Autodesk Inventor part; units mm, degrees
ref_plane "Start Plane" through (0, 0, -31.4468) normal (0, 0, 1) x (1, 0, 0)
ref_plane "End Plane" through (0, 0, 1160.255) normal (0, 0, 1) x (1, 0, 0)
ref_plane "Work Plane4" through (-6.5041, 0, 1155.5322) normal (0.2588, 0, 0.9659) x (0.9659, 0, -0.2588)
ref_plane "Start Plane" through (0, 0, -31.4468) normal (0, 0, 1) x (1, 0, 0)
ref_plane "End Plane" through (0, 0, 1160.255) normal (0, 0, 1) x (1, 0, 0)
sketch "Sketch" plane through (0, 0, 0) normal (0, 0, 1) x (1, 0, 0)
  circle A0 centre (0, 0) radius 20.447
  circle A1 centre (0, 0) radius 24.13
  dimension "d0" = 48.26
  dimension "d1" = 3.683
extrude "Body" add sketch "Sketch" along normal up to surface (1191.7019 mm away) from surface at -31.4468
sketch "Sketch3" plane through (0, 0, 0) normal (0, 0, 1) x (1, 0, 0)
  line L0 (0, 0) -> (10, 0)
ref_plane "Work Plane3" through (0, 0, 0) normal (0, -1, 0) x (1, 0, 0)
ref_plane "Work Plane4" through (-6.5041, 0, 1155.5322) normal (0.2588, 0, 0.9659) x (0.9659, 0, -0.2588)
split "Split1" plane through (-6.5041, 0, 1155.5322) removes the side toward (0.2588, 0, 0.9659)
ref_plane "Work Plane5" through (-982.5186, 0, 238.2838) normal (-0.2588, 0, -0.9659) x (-0.9659, 0, 0.2588)
split "Split2" plane through (-982.5186, 0, 238.2838) removes the side toward (-0.2588, 0, -0.9659)
sketch "Sketch4" plane through (0, 0, 0) normal (0, -1, 0) x (1, 0, 0)
  line L0 (-2, -31.4468) -> (12, -31.4468)
  line L1 (-2, 1160.255) -> (12, 1160.255)
  dimension "d7" = 1191.7018
equation "\"d0\" = G_H"
equation "\"d1\" = G_T"
equation "\"d2\" = G_L"
equation "\"G_H\" = 48.26"
equation "\"G_T\" = 3.683"
equation "\"G_L\" = d7"
equation "\"G_OFFSET_START\" = 31.44683"
equation "\"G_OFFSET_END\" = -19.55088"
equation "\"d4\" = -G_OFFSET_START"
equation "\"d5\" = G_OFFSET_END + B_L"
equation "\"B_L\" = 1179.8059"
properties part number "ANSI - 1 1/2 x 0.145 - 46.917" material "Steel, Mild"
Design review of the part built by this model. Coordinates are the model's own, in mm. Coordinates: 2 decimals unless noted, no trailing zeros. Write each loop counter-clockwise with the first axis right and the second up, starting at its lowest first coordinate (ties: lowest second). Pieces come first, ordered by that corner, then holes.
1) Mouldability with a two-part tool opening along Y and no side actions: class faces 1 (the cylindrical face through (23.016, -7.248, 556.106)), 2 (the cylindrical face through (-16.226, 12.442, 556.112)), 3 (the flat face through (-10.837, 17.987, -22.077)) as +Y half, -Y half, draft (parallel to the pull), parting line (faces both ways), or undercut.
2) Insertion check: pin 1 (4 mm diameter, centred on x = -18, z = 636.5, fed in from -Y); pin 2 (1.5 mm diameter, centred on x = -11.5, z = 329.5, fed in from -Y); pin 3 (6 mm diameter, centred on x = -18, y = 16.5, fed in from -Z). Each pin has a flat end and moves straight along its axis. Give the tip position at first contact, or say it passes through.
3) To check wall thickness, follow L1, parallel to X at y = 0, z = 497; L2, parallel to Y at x = 2, z = 502. State the ranges of each line that lie inside material, in increasing order.
4) Add section B-B (y = 7.5). Write out the cut boundary in (x, z), plus the area to 3 significant figures.
5) Add section A-A (x = 0). Write out the cut boundary in (y, z), plus the area to 3 significant figures.
6) Add section C-C (z = 577). Write out the cut boundary in (x, y).
Check result:
1. face 1: parting line
1. face 2: undercut
1. face 3: draft
2. pin 1: stops at y = -18.06
2. pin 2: stops at y = -21.6
2. pin 3: stops at z = -20.96
3. L1: x = -24.13 to -20.45, 20.45 to 24.13
3. L2: y = -24.05 to -20.35, 20.35 to 24.05
4. outline: (-22.93, -18.84) - (-19.02, -19.88) - (-19.02, 1158.89) - (-22.93, 1159.93) - close; (19.02, -30.08) - (22.93, -31.13) - (22.93, 1147.64) - (19.02, 1148.69) - close
4. area: 9,230 mm2
5. outline: (-24.13, -24.98) - (-20.45, -24.98) - (-20.45, 1153.79) - (-24.13, 1153.79) - close; (20.45, -24.98) - (24.13, -24.98) - (24.13, 1153.79) - (20.45, 1153.79) - close
5. area: 8,680 mm2
6. outline: circle Ø48.26 at (0, 0); hole circle Ø40.89 at (0, 0)
